Geometry: final body of the model. Coordinates: model frame, mm. A direction names the side the tool comes from. Give positions to 0.01 mm unless a question says otherwise; leave off trailing zeros. Order: outer loops, then holes, each group sorted by start corner. A loop starts at its lowest first (then second) coordinate and runs counter-clockwise, first axis right, second up. Notation, with made-up numbers: M 58.5,25 L 74.5,25 A16 cw 74.5,51 Z; hole C -25,-16.75 d5. An arc over 180 degrees is marked long. Use CSV: the item, a comma, the result in double quotes.
```python
from build123d import *

# Parameters (mm, degrees)
SKETCH1_W           = 17.4
SKETCH1_H           = 38.4
BOSS_EXTRUDE1_DEPTH = 6.5
FILLET1_R           = 3.5
CUT_EXTRUDE1_DEPTH  = 5
SKETCH3_R           = 4
SKETCH3_R_2         = 2.75
BOSS_EXTRUDE2_DEPTH = 4.8
SKETCH4_R           = 2.75
CUT_EXTRUDE2_DEPTH  = 0.9


with BuildPart() as part:
    # Sketch1 → Boss-Extrude1 (new body)
    with BuildSketch(Plane(origin=(0, 0, 0), x_dir=(1, 0, 0), z_dir=(0, 1, 0))):
        with Locations((-8.7, -19.2)):
            Rectangle(SKETCH1_W, SKETCH1_H)
    extrude(amount=BOSS_EXTRUDE1_DEPTH)

    # Fillet1
    fillet1_edges = [part.edges().sort_by_distance(p)[0] for p in [
        (0, 3.25, 38.4),
        (-17.4, 3.25, 38.4),
        (-17.4, 3.25, 0),
        (0, 3.25, 0),
    ]]
    fillet(fillet1_edges, radius=FILLET1_R)

    # Sketch2 → Cut-Extrude1 (cut)
    with BuildSketch(Plane(origin=(0, 6.5, 0), x_dir=(1, 0, 0), z_dir=(0, 1, 0))):
        with BuildLine():
            Line((-13.9, -36.9), (-3.5, -36.9))
            ThreePointArc((-3.5, -36.9), (-2.085786438, -36.314213562), (-1.5, -34.9))
            Line((-1.5, -34.9), (-1.5, -3.5))
            ThreePointArc((-1.5, -3.5), (-2.085786438, -2.085786438), (-3.5, -1.5))
            Line((-3.5, -1.5), (-13.9, -1.5))
            ThreePointArc((-13.9, -1.5), (-15.314213562, -2.085786438), (-15.9, -3.5))
            Line((-15.9, -3.5), (-15.9, -34.9))
            ThreePointArc((-15.9, -34.9), (-15.314213562, -36.314213562), (-13.9, -36.9))
        make_face()
    extrude(amount=-CUT_EXTRUDE1_DEPTH, mode=Mode.SUBTRACT)

    # Sketch3 → Boss-Extrude2 (add)
    with BuildSketch(Plane(origin=(0, 1.5, 0), x_dir=(1, 0, 0), z_dir=(0, 1, 0))):
        with Locations((-8.7, -29.7)):
            Circle(SKETCH3_R)
        with Locations((-8.7, -29.7)):
            Circle(SKETCH3_R_2, mode=Mode.SUBTRACT)
        with Locations((-8.7, -8.7)):
            Circle(SKETCH3_R)
        with Locations((-8.7, -8.7)):
            Circle(SKETCH3_R_2, mode=Mode.SUBTRACT)
    extrude(amount=BOSS_EXTRUDE2_DEPTH)

    # Sketch4 → Cut-Extrude2 (cut)
    with BuildSketch(Plane(origin=(0, 1.5, 0), x_dir=(1, 0, 0), z_dir=(0, 1, 0))):
        with Locations((-8.7, -29.7)):
            Circle(SKETCH4_R)
        with Locations((-8.7, -8.7)):
            Circle(SKETCH4_R)
    extrude(amount=-CUT_EXTRUDE2_DEPTH, mode=Mode.SUBTRACT)


solid = part.part
```
1. Pin query (flat end, axial travel): pin 1 Ø2.5 at (x, z) = (-8, 8) entering from +Y; pin 2 Ø7 at (x, z) = (-8.7, 8.7) entering from +Y; pin 3 Ø4 at (x, z) = (-10.5, 10) entering from -Y; pin 4 Ø1 at (x, z) = (-13.5, 26) entering from +Y. Return the tip coordinate at first contact, or that it passes through.
Answer:
pin 1,"y = 0.6"
pin 2,"y = 6.3"
pin 3,"y = 0"
pin 4,"y = 1.5"
2. Section A-A, the plane y = 2.25. Return the cut outline in (x, z).
Answer:
outline,"M -17.4,3.5 A3.5 ccw -13.9,0 L -3.5,0 A3.5 ccw 0,3.5 L 0,34.9 A3.5 ccw -3.5,38.4 L -13.9,38.4 A3.5 ccw -17.4,34.9 Z; C -8.7,8.7 d8; C -8.7,29.7 d8; hole M -15.9,3.5 A2 ccw -13.9,1.5 L -3.5,1.5 A2 ccw -1.5,3.5 L -1.5,34.9 A2 ccw -3.5,36.9 L -13.9,36.9 A2 ccw -15.9,34.9 Z; hole C -8.7,8.7 d5.5; hole C -8.7,29.7 d5.5"
3. Line query: line 1 (X direction, y = 2.85, z = 8.7); line 2 (Z direction, x = -8.7, y = 1.95); line 3 (Z direction, x = -4.5, y = 4). Output: solid intervals per line, ascending.
Answer:
line 1,"-17.4 to -15.9, -12.7 to -11.45, -5.95 to -4.7, -1.5 to 0"
line 2,"0 to 1.5, 4.7 to 5.95, 11.45 to 12.7, 25.7 to 26.95, 32.45 to 33.7, 36.9 to 38.4"
line 3,"0 to 1.5, 36.9 to 38.4"
4. Section D-D, the plane z = 29.7. Return the cut outline in (x, y), plus the area to 4 significant figures.
Answer:
outline,"M -17.4,0 L 0,0 L 0,6.5 L -1.5,6.5 L -1.5,1.5 L -4.7,1.5 L -4.7,6.3 L -5.95,6.3 L -5.95,0.6 L -11.45,0.6 L -11.45,6.3 L -12.7,6.3 L -12.7,1.5 L -15.9,1.5 L -15.9,6.5 L -17.4,6.5 Z"
area,"48.15 mm2"
5. Section B-B, the plane x = -8.7. Return the cut outline in (y, z).
Answer:
outline,"M 0,0 L 6.5,0 L 6.5,1.5 L 1.5,1.5 L 1.5,4.7 L 6.3,4.7 L 6.3,5.95 L 0.6,5.95 L 0.6,11.45 L 6.3,11.45 L 6.3,12.7 L 1.5,12.7 L 1.5,25.7 L 6.3,25.7 L 6.3,26.95 L 0.6,26.95 L 0.6,32.45 L 6.3,32.45 L 6.3,33.7 L 1.5,33.7 L 1.5,36.9 L 6.5,36.9 L 6.5,38.4 L 0,38.4 Z"
6. Pull-direction query (X, two-part tool) for faces 1 (the face through (-16.4, 3.3, 37.35)), 2 (the face through (-9, 0, 19)), 3 (the face through (-15.9, 4, 19)); classes: +X half, -X half, draft (parallel to the pull), parting line (faces both ways), or undercut.
Answer:
face 1,"-X half"
face 2,"draft"
face 3,"undercut"
7. Reachability of faces 4 (the face through (-10, 6.3, 27)), 5 (the face through (-1, 3.3, 1.05)) from +Z, -Z, +X, -X, +Y, -Y: full face, straight path, thin tool, end or side. Return the list, or none.
Answer:
face 4,"+Y"
face 5,"-Z, +X, +Y, -Y"
8. Section C-C, the plane z = 20. Return the cut outline in (x, y), plus the area to 3 significant figures.
Answer:
outline,"M -17.4,0 L 0,0 L 0,6.5 L -1.5,6.5 L -1.5,1.5 L -15.9,1.5 L -15.9,6.5 L -17.4,6.5 Z"
area,"41.1 mm2"
